```python
from build123d import *

# Parameters (mm, degrees)
BOSS_EXTRUDE3_DEPTH      = 4
BOSS_EXTRUDE4_DEPTH      = 4
BOSS_EXTRUDE4_DEPTH_BACK = 1
SKETCH2_6_W              = 12
SKETCH2_6_H              = 12
BOSS_EXTRUDE5_DEPTH      = 14
SKETCH3_R                = 2.5
CUT_EXTRUDE1_DEPTH       = 14


with BuildPart() as part:
    # Sketch2 → Boss-Extrude3 (new body)
    with BuildSketch(Plane(origin=(0, 0, 0), x_dir=(1, 0, 0), z_dir=(0, 1, 0))):
        with BuildLine():
            ThreePointArc((5.818261974, 15.438591174), (2.165693386, 14.198711204), (0.022707007, 10.991505409))
            ThreePointArc((0.022707007, 10.991505409), (1.058141943, 5.786022585), (5.818261974, 3.438591174))
            Line((5.818261974, 3.438591174), (10.422223902, 3.438591174))
            Line((10.422223902, 3.438591174), (13.637614211, 15.438591174))
            Line((13.637614211, 15.438591174), (5.818261974, 15.438591174))
        make_face()
        with BuildLine():
            Line((11.441310363, 53.606313284), (0.022707007, 10.991505409))
            ThreePointArc((0.022707007, 10.991505409), (2.165693386, 14.198711204), (5.818261974, 15.438591174))
            Line((5.818261974, 15.438591174), (13.637614211, 15.438591174))
            Line((13.637614211, 15.438591174), (23.032420278, 50.500484743))
            ThreePointArc((23.032420278, 50.500484743), (15.68395105, 46.257844056), (11.441310363, 53.606313284))
        make_face()
        Polygon((13.637614211, 15.438591174), (10.422223902, 3.438591174), (93.119532163, 3.438591174), (93.119532163, 15.438591174), align=None)
        with BuildLine():
            Line((0.022707007, 10.991505409), (-6.676022794, -14.008494556))
            ThreePointArc((-6.676022794, -14.008494556), (-0.097310683, -9.612739658), (5.119532163, -15.561408826))
            ThreePointArc((5.119532163, -15.561408826), (5.068201332, -16.34456598), (4.915087121, -17.114323097))
            Line((4.915087121, -17.114323097), (10.422223902, 3.438591174))
            Line((10.422223902, 3.438591174), (5.818261974, 3.438591174))
            ThreePointArc((5.818261974, 3.438591174), (1.058141943, 5.786022585), (0.022707007, 10.991505409))
        make_face()
        with BuildLine():
            Line((105.119532163, 15.438591174), (105.119532163, 3.438591174))
            Line((105.119532163, 3.438591174), (139.119532163, 3.438591174))
            ThreePointArc((139.119532163, 3.438591174), (133.119532163, 9.438591174), (139.119532163, 15.438591174))
            Line((139.119532163, 15.438591174), (105.119532163, 15.438591174))
        make_face()
    extrude(amount=BOSS_EXTRUDE3_DEPTH)

    # Sketch2_5 → Boss-Extrude4 (add, two sides)
    with BuildSketch(Plane(origin=(0, 0, 0), x_dir=(1, 0, 0), z_dir=(0, 1, 0))) as boss_extrude4_sk:
        with BuildLine():
            ThreePointArc((5.119532163, -15.561408826), (-0.097310683, -9.612739658), (-6.676022794, -14.008494556))
            ThreePointArc((-6.676022794, -14.008494556), (-2.433382107, -21.356963784), (4.915087121, -17.114323097))
            ThreePointArc((4.915087121, -17.114323097), (5.068201332, -16.34456598), (5.119532163, -15.561408826))
        make_face()
        with BuildLine():
            ThreePointArc((23.236865321, 52.053399014), (18.020022474, 58.002068182), (11.441310363, 53.606313284))
            ThreePointArc((11.441310363, 53.606313284), (15.68395105, 46.257844056), (23.032420278, 50.500484743))
            ThreePointArc((23.032420278, 50.500484743), (23.185534489, 51.27024186), (23.236865321, 52.053399014))
        make_face()
        with BuildLine():
            ThreePointArc((139.119532163, 15.438591174), (133.119532163, 9.438591174), (139.119532163, 3.438591174))
            ThreePointArc((139.119532163, 3.438591174), (143.362172851, 5.195950486), (145.119532163, 9.438591174))
            ThreePointArc((145.119532163, 9.438591174), (143.362172851, 13.681231861), (139.119532163, 15.438591174))
        make_face()
    extrude(amount=BOSS_EXTRUDE4_DEPTH)
    extrude(boss_extrude4_sk.sketch, amount=-BOSS_EXTRUDE4_DEPTH_BACK)

    # Sketch2_6 → Boss-Extrude5 (add)
    with BuildSketch(Plane(origin=(0, 0, 0), x_dir=(1, 0, 0), z_dir=(0, 1, 0))):
        with Locations((99.119532163, 9.438591174)):
            Rectangle(SKETCH2_6_W, SKETCH2_6_H)
    extrude(amount=BOSS_EXTRUDE5_DEPTH)

    # Sketch3 → Cut-Extrude1 (cut)
    with BuildSketch(Plane.XY.offset(-3.438591174)):
        with Locations((99.119532163, 14)):
            Circle(SKETCH3_R)
    extrude(amount=-CUT_EXTRUDE1_DEPTH, mode=Mode.SUBTRACT)


solid = part.part
```
Verification items for the finished model (mm, model axes). A direction names the side the tool comes from. Give positions to 0.01 mm unless a question says otherwise; leave off trailing zeros. Loops run counter-clockwise (first coordinate to the right, second up) from the corner with the lowest first, then second, coordinate; pieces in that order, holes last.
1. Thickness scan on line 1 (Z direction, x = 86.5, y = 1.5); line 2 (Y direction, x = 7, z = -32.5); line 3 (X direction, y = 9.75, z = -13.5). Record the ranges inside material, lowest first.
2. Section check B-B, the plane y = 2.5. Enter the section's corners in (x, z).
3. Section check A-A, the plane x = 16. Enter the section's corners in (y, z), then the cut area to 3 significant figures.
4. Section check D-D, the plane x = 43. Enter the section's corners in (y, z), then the cut area to 3 significant figures.
5. Mould release check, pull along Z, two halves, no side actions. Record for faces 1 (the flat face through (17, -1, -52)), 2 (the flat face through (7.63, 1.97, 6.98)), 3 (the flat face through (18.27, 1.97, -32.72)): released by +Z, released by -Z, zero draft, split by the parting line, or undercut.
6. Section check C-C, the plane z = -8. Enter the section's corners in (x, y).
7. Go/stop test with flat-tipped pins: pin 1 Ø13 at (x, z) = (132, -7.5) entering from +Y; pin 2 Ø7 at (x, y) = (66, 5.5) entering from +Z; pin 3 Ø7 at (x, y) = (54.5, 7) entering from -Z; pin 4 Ø3 at (x, y) = (53.5, 6.5) entering from +Z. Record where each tip stops, or that it passes through.
8. Set-up check for faces 4 (the cylindrical face through (18.022, 0.909, -58.002)), 5 (the flat face through (93.12, 9, -9)), 6 (the flat face through (125, 4, -10)), 7 (the flat face through (95, 14, -10)), 8 (the flat face through (73.9, 3.8, -3.439)): record each of +Z, -Z, +X, -X, +Y, -Y from which the full face is reachable in a straight line by a thin tool's end or side.
Geometry says:
1. line 1: z = -15.44 to -3.44
1. line 2: y = 0 to 4
1. line 3: x = 93.12 to 105.12
2. outline: (-6.68, 14.01) - (11.44, -53.61) arc R6 ccw to (23.03, -50.5) - (13.64, -15.44) - (139.12, -15.44) arc R6 ccw to (139.12, -3.44) - (10.42, -3.44) - (4.92, 17.11) arc R6 ccw to start
3. outline: (-1, -57.92) - (4, -57.92) - (4, -24.26) - (0, -24.26) - (0, -46.18) - (-1, -46.18) - close; (0, -15.44) - (4, -15.44) - (4, -3.44) - (0, -3.44) - close
3. area: 194 mm2
4. outline: (0, -15.44) - (4, -15.44) - (4, -3.44) - (0, -3.44) - close
4. area: 48.0 mm2
5. face 1: zero draft
5. face 2: released by +Z
5. face 3: undercut
6. outline: (-0.78, 0) - (133.29, 0) - (133.29, -1) - (144.94, -1) - (144.94, 4) - (105.12, 4) - (105.12, 14) - (101.62, 14) arc R2.5 cw to (96.62, 14) - (93.12, 14) - (93.12, 4) - (-0.78, 4) - close
7. pin 1: stops at y = 4
7. pin 2: stops at z = -3.44
7. pin 3: stops at z = -15.44
7. pin 4: passes through
8. face 4: -Y
8. face 5: +Z, -Z, -X, +Y
8. face 6: +Z, -Z, +X, +Y
8. face 7: +Z, -Z, +X, -X, +Y
8. face 8: +Z, +X, +Y, -Y
